Geometry check sheet. Reference: the model listing, model coordinates, mm. A direction names the side the tool comes from. Round coordinates to 2 decimals unless told otherwise and drop trailing zeros. Order: outer loops, then holes, each group sorted by start corner. A loop starts at its lowest first (then second) coordinate and runs counter-clockwise, first axis right, second up. Notation, with made-up numbers: (-20, 11.5) -> (2, 11.5) arc R10 ccw to (2, 28.5) -> close; hole circle Ø5 at (-32.75, -14.75). An arc over 180 degrees is marked (long way). Use a Markdown table: item, result. Add a question column.
Item 1: Mould release check, pull along X, two halves, no side actions. Record for faces 1 (the cylindrical face through (0.76, -25.7, 43.15)), 2 (the cylindrical face through (-56.7, -11.8, -43.1)), 3 (the flat face through (-54.2, -11, -1)), 4 (the flat face through (-1, -23.25, 1)): pulls with the +X half, pulls with the -X half, needs draft (parallel to the pull), parting line crosses it, or undercut.
Item 2: Sectioned sample at C-C, the plane z = 37. Record the cut outline in (x, y), and give its area (3 significant figures).
Item 3: Sectioned sample at B-B, the plane x = -47. Record the cut outline in (y, z).
Item 4: Gauge pin test, flat end, axial feed: pin 1 Ø24.5 at (x, z) = (3.5, -15) entering from +Y. Record the tip position at first contact, or that the pin passes through.
Item 5: Set-up check for faces 5 (the flat face through (-1, -11, -40.65)), 6 (the cylindrical face through (0.76, -25.7, -43.15)): record each of +Z, -Z, +X, -X, +Y, -Y from which the full face is reachable in a straight line by a thin tool's end or side.
Item 6: Material ranges on probe 1 along Z at (x, y) = (51, -2.5); probe 2 along X at (y, z) = (-5.5, 21); probe 3 along Y at (x, z) = (30.5, -28), recorded low to high. Write a range as [from, to].
Item 7: Sectioned sample at A-A, the plane y = -16.5. Record the cut outline in (x, z), and give its area (3 significant figures).
from build123d import *

# Parameters (mm, degrees)
SKETCH_W    = 108.4
SKETCH_H    = 81.3
PAD_DEPTH   = 23.25
THICKNESS_T = 3.5


with BuildPart() as part:
    # Sketch → Pad (new body)
    with BuildSketch(Plane.XZ):
        Rectangle(SKETCH_W, SKETCH_H)
    extrude(amount=PAD_DEPTH)

    # Thickness
    thickness_openings = [part.faces().sort_by_distance(p)[0] for p in [
        (0, 0, 0),
    ]]
    offset(amount=THICKNESS_T, openings=thickness_openings)


solid = part.part
Found:
| question | item | result |
|---|---|---|
| 1 | face 1 | needs draft |
| 1 | face 2 | pulls with the -X half |
| 1 | face 3 | undercut |
| 1 | face 4 | undercut |
| 2 | outline | (-57.7, -23.25) arc R3.5 ccw to (-54.2, -26.75) -> (54.2, -26.75) arc R3.5 ccw to (57.7, -23.25) -> (57.7, 0) -> (54.2, 0) -> (54.2, -23.25) -> (-54.2, -23.25) -> (-54.2, 0) -> (-57.7, 0) -> close |
| 2 | area | 561 mm2 |
| 3 | outline | (-26.75, -40.65) arc R3.5 ccw to (-23.25, -44.15) -> (0, -44.15) -> (0, -40.65) -> (-23.25, -40.65) -> (-23.25, 40.65) -> (0, 40.65) -> (0, 44.15) -> (-23.25, 44.15) arc R3.5 ccw to (-26.75, 40.65) -> close |
| 4 | pin 1 | stops at y = -23.25 |
| 5 | face 5 | +Y |
| 5 | face 6 | -Z, +X, -X, -Y |
| 6 | probe 1 | z = [-44.15, -40.65], [40.65, 44.15] |
| 6 | probe 2 | x = [-57.7, -54.2], [54.2, 57.7] |
| 6 | probe 3 | y = [-26.75, -23.25] |
| 7 | outline | (-57.7, -40.65) arc R3.5 ccw to (-54.2, -44.15) -> (54.2, -44.15) arc R3.5 ccw to (57.7, -40.65) -> (57.7, 40.65) arc R3.5 ccw to (54.2, 44.15) -> (-54.2, 44.15) arc R3.5 ccw to (-57.7, 40.65) -> close; hole (-54.2, -40.65) -> (54.2, -40.65) -> (54.2, 40.65) -> (-54.2, 40.65) -> close |
| 7 | area | 1,370 mm2 |
